Source: three-view drawing plus pictorial views. Frame: mm from the lowest corner of the part. A direction names the side the tool comes from. Give positions to 0.01 mm unless a question says otherwise; leave off trailing zeros. Write each loop counter-clockwise with the first axis right and the second up, starting at its lowest first coordinate (ties: lowest second). Pieces come first, ordered by that corner, then holes. Notation, with made-up numbers: (72, 35.5) -> (127, 35.5) arc R15 ccw to (127, 50.5) -> close; hole circle Ø5 at (23, -7.5). An arc over 180 degrees is marked (long way). Answer in a Markdown table with one row per item. Add a question column.
Item 1: Material intervals for probe 1 along X at (y, z) = (6, 8.5) (1 decimal); probe 2 along X at (y, z) = (5.75, 35.5) (1 decimal); probe 3 along X at (y, z) = (1.75, 23) (1 decimal), sorted ascending. Write a range as from..to.
Item 2: Section query C-C on y = 7.25. State how many separate pieces and enclosed holes the cut face has, plus the area to 3 significant figures.
Item 3: Section query D-D on z = 9. Output: boundary loops of the cut face in (x, y) (1 decimal).
Item 4: Section query A-A on z = 24. Output: boundary loops of the cut face in (x, y), plus the area to 3 significant figures.
Item 5: Draft query along Z for the marked faces 4, 5 and 6. Return one class per face: +Z half, -Z half, draft (parallel to the pull), parting line (faces both ways), or undercut.
Item 6: First-contact query: P1, Ø1, axis at y = 8, z = 11.5, coming from the +X side (1 decimal); P2, Ø6, axis at y = 4, z = 24.5, coming from the +X side; P3, Ø4, axis at x = 20.5, z = 10, coming from the -Y side; P4, Ø3.5, axis at x = 24, z = 24, coming from the +Y side. Flat tips, straight axial feed; report the tip coordinate or a pass-through.
Item 7: Section query B-B on x = 24. Output: boundary loops of the cut face in (y, z), plus the area to 3 significant figures.
Item 8: Access query for the marked faces 1, 2 and 3. Directions: +Z, -Z, +X, -X, +Y, -Y. A direction counts if a zero-diameter tool reaches every point of the face in a straight line with its end or side. Return the directions, or none.
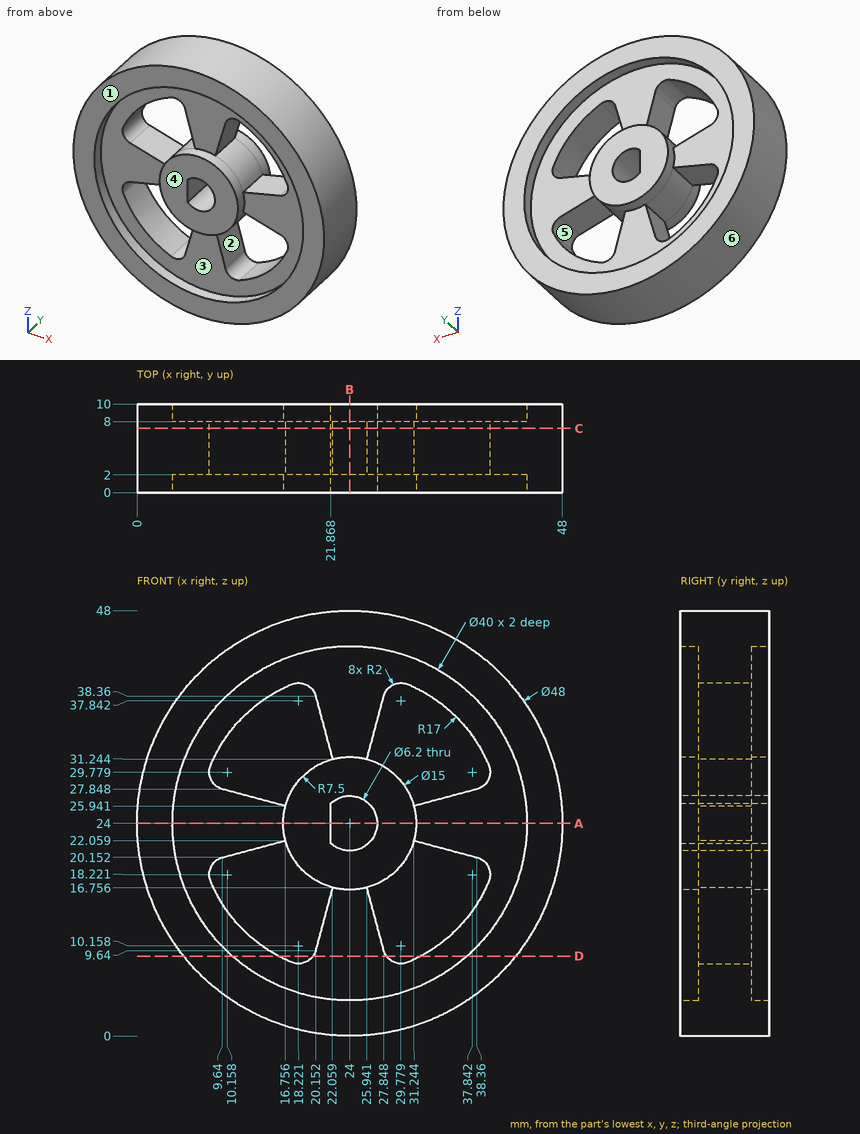
Findings below:
| question | item | result |
|---|---|---|
| 1 | probe 1 | x = 5.7..17, 19.3..28.7, 31..42.3 |
| 1 | probe 2 | x = 2.9..11.5, 20.9..27.1, 36.5..45.1 |
| 1 | probe 3 | x = 0..4, 16.6..21.9, 26.9..31.4, 44..48 |
| 2 | separate pieces | 1 |
| 2 | enclosed holes | 5 |
| 2 | area | 1,300 mm^2 |
| 3 | outline | (5.3, 0) -> (10.8, 0) -> (10.8, 2) -> (16, 2) -> (16, 8) -> (10.8, 8) -> (10.8, 10) -> (5.3, 10) -> close; (19.9, 2) -> (28.1, 2) -> (28.1, 8) -> (19.9, 8) -> close; (32, 2) -> (37.2, 2) -> (37.2, 0) -> (42.7, 0) -> (42.7, 10) -> (37.2, 10) -> (37.2, 8) -> (32, 8) -> close |
| 4 | outline | (0, 0) -> (4, 0) -> (4, 2) -> (16.5, 2) -> (16.5, 0) -> (21.87, 0) -> (21.87, 10) -> (16.5, 10) -> (16.5, 8) -> (4, 8) -> (4, 10) -> (0, 10) -> close; (27.1, 0) -> (31.5, 0) -> (31.5, 2) -> (44, 2) -> (44, 0) -> (48, 0) -> (48, 10) -> (44, 10) -> (44, 8) -> (31.5, 8) -> (31.5, 10) -> (27.1, 10) -> close |
| 4 | area | 328 mm^2 |
| 5 | face 4 | draft |
| 5 | face 5 | undercut |
| 5 | face 6 | parting line |
| 6 | P1 | stops at x = 44.8 |
| 6 | P2 | stops at x = 48 |
| 6 | P3 | stops at y = 2 |
| 6 | P4 | passes through |
| 7 | outline | (0, 0) -> (10, 0) -> (10, 4) -> (8, 4) -> (8, 16.5) -> (10, 16.5) -> (10, 20.9) -> (0, 20.9) -> (0, 16.5) -> (2, 16.5) -> (2, 4) -> (0, 4) -> close; (0, 27.1) -> (10, 27.1) -> (10, 31.5) -> (8, 31.5) -> (8, 44) -> (10, 44) -> (10, 48) -> (0, 48) -> (0, 44) -> (2, 44) -> (2, 31.5) -> (0, 31.5) -> close |
| 7 | area | 318 mm^2 |
| 8 | face 1 | +Z, -Z, +X, -X, -Y |
| 8 | face 2 | +Y, -Y |
| 8 | face 3 | -Y |
